```python
from build123d import *

# Parameters (mm, degrees)
SKETCH_1_W          = 35
SKETCH_1_H          = 19
SKETCH_1_R          = 2.1
EXTRUDE_1_DEPTH     = 6
SKETCH_2_W          = 19
SKETCH_2_H          = 19
EXTRUDE_2_DEPTH     = 64
SKETCH_4_R          = 1.5
CUT_EXTRUDE_1_DEPTH = 10


with BuildPart() as part:
    # 草图1 → 凸台-拉伸1 (new body)
    with BuildSketch(Plane(origin=(0, 0, 0), x_dir=(1, 0, 0), z_dir=(0, 1, 0))):
        Rectangle(SKETCH_1_W, SKETCH_1_H)
        with Locations(Location((-11.5, 0, 0), (0, 0, 270))):
            Circle(SKETCH_1_R, mode=Mode.SUBTRACT)
    extrude(amount=EXTRUDE_1_DEPTH)

    # 草图2 → 凸台-拉伸2 (add)
    with BuildSketch(Plane(origin=(0, 6, 0), x_dir=(1, 0, 0), z_dir=(0, 1, 0))):
        with Locations((8, 0)):
            Rectangle(SKETCH_2_W, SKETCH_2_H)
    extrude(amount=EXTRUDE_2_DEPTH)

    # 草图4 → 切除-拉伸1 (cut)
    with BuildSketch(Plane(origin=(0, 70, 0), x_dir=(1, 0, 0), z_dir=(0, 1, 0))):
        with Locations(Location((8, 0, 0), (0, 0, 270))):
            Circle(SKETCH_4_R)
    extrude(amount=-CUT_EXTRUDE_1_DEPTH, mode=Mode.SUBTRACT)


solid = part.part
```
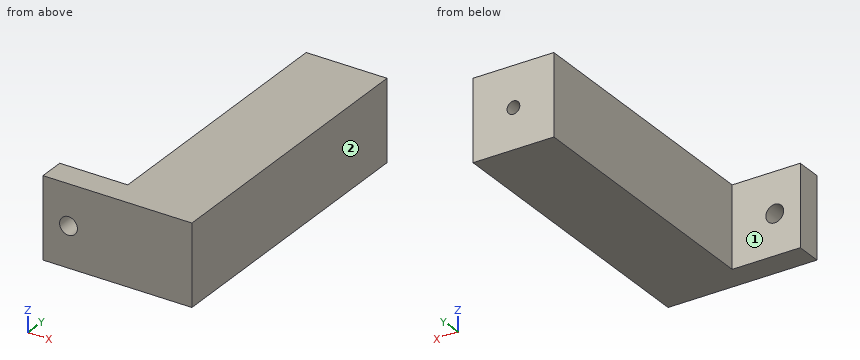
CAD build for the part. Positions are in the model's coordinates, mm. Face numbers are marked on the shaded views. A direction names the side the tool comes from. Round coordinates to 2 decimals unless told otherwise and drop trailing zeros. Write each loop counter-clockwise with the first axis right and the second up, starting at its lowest first coordinate (ties: lowest second). Pieces come first, ordered by that corner, then holes. Notation, with made-up numbers: (-1, 75) - (29, 75) arc R33 ccw to (29, 109) - close; hole circle Ø11 at (-4.75, 68). An arc over 180 degrees is marked (long way). Write item = value, one per line. Start each with the question number.
Q1. Band-saw the part on A-A (z = 0). Give the cut face in (x, y), then the cut area to 3 significant figures.
Q2. Band-saw the part on B-B (x = -11.5). Give the cut face in (y, z).
Q3. Band-saw the part on C-C (z = 5.25). Give the cut face in (x, y), then the cut area to 3 significant figures.
Q4. Drop flat-ended pins along their axis: pin 1 (1 mm diameter, centred on x = -12, z = -6.5, fed in from -Y); pin 2 (9.5 mm diameter, centred on y = 45, z = 2, fed in from -X); pin 3 (1.5 mm diameter, centred on x = 8.5, z = 0.5, fed in from +Y). Give the stop position or say it passes through.
Q5. Which spindle directions (+Z, -Z, +X, -X, +Y, -Y) get a long thin tool onto all of the face, cutting with end or side? Do the marked faces 1 and 2. Say none if no direction does.
Q6. Probe L1, parallel to X at y = 1.8, z = 0; L2, parallel to X at y = 63.75, z = 0; L3, parallel to X at y = 41.5, z = 7. List the from-to ranges inside material, lowest first. Write a range as from..to.
Q7. Band-saw the part on D-D (x = 8). Give the cut face in (y, z), then the cut area to 3 significant figures.
Answers below:
q1.outline = (-17.5, 0) - (-13.6, 0) - (-13.6, 6) - (-17.5, 6) - close; (-9.4, 0) - (17.5, 0) - (17.5, 70) - (9.5, 70) - (9.5, 60) - (6.5, 60) - (6.5, 70) - (-1.5, 70) - (-1.5, 6) - (-9.4, 6) - close
q1.area = 1,370 mm2
q2.outline = (0, -9.5) - (6, -9.5) - (6, -2.1) - (0, -2.1) - close; (0, 2.1) - (6, 2.1) - (6, 9.5) - (0, 9.5) - close
q3.outline = (-17.5, 0) - (17.5, 0) - (17.5, 70) - (-1.5, 70) - (-1.5, 6) - (-17.5, 6) - close
q3.area = 1,430 mm2
q4.pin_1 = 0
q4.pin_2 = -1.5
q4.pin_3 = 60
q5.face_1 = +Z, -Z, -X, +Y
q5.face_2 = +Z, -Z, +X, +Y, -Y
q6.L1 = -17.5..-13.6, -9.4..17.5
q6.L2 = -1.5..6.5, 9.5..17.5
q6.L3 = -1.5..17.5
q7.outline = (0, -9.5) - (70, -9.5) - (70, -1.5) - (60, -1.5) - (60, 1.5) - (70, 1.5) - (70, 9.5) - (0, 9.5) - close
q7.area = 1,300 mm2
